from build123d import *

# Parameters (mm, degrees)
SKETCH1_R           = 32.5
BOSS_EXTRUDE1_DEPTH = 6
SKETCH16_R          = 1.1
CUT_EXTRUDE8_DEPTH  = 7
SKETCH17_R          = 2
CUT_EXTRUDE9_DEPTH  = 2.4
SKETCH12_R          = 1.65
CUT_EXTRUDE10_DEPTH = 7
CUT_EXTRUDE11_DEPTH = 3
CUT_EXTRUDE12_DEPTH = 7


with BuildPart() as part:
    # Sketch1 → Boss-Extrude1 (new body)
    with BuildSketch(Plane.XY):
        Circle(SKETCH1_R)
    extrude(amount=BOSS_EXTRUDE1_DEPTH)

    # Sketch16 → Cut-Extrude8 (cut, through all)
    with BuildSketch(Plane.XY.offset(6)):
        with Locations((8, 0)):
            Circle(SKETCH16_R)
        with Locations((-8, 0)):
            Circle(SKETCH16_R)
        with Locations((0, -8)):
            Circle(SKETCH16_R)
        with Locations((0, 8)):
            Circle(SKETCH16_R)
    extrude(amount=-CUT_EXTRUDE8_DEPTH, mode=Mode.SUBTRACT)

    # Sketch17 → Cut-Extrude9 (cut)
    with BuildSketch(Plane.XY.offset(6)):
        with Locations((8, 0)):
            Circle(SKETCH17_R)
        with Locations((-8, 0)):
            Circle(SKETCH17_R)
        with Locations((0, -8)):
            Circle(SKETCH17_R)
        with Locations((0, 8)):
            Circle(SKETCH17_R)
    extrude(amount=-CUT_EXTRUDE9_DEPTH, mode=Mode.SUBTRACT)

    # Sketch12 → Cut-Extrude10 (cut, through all)
    with BuildSketch(Plane.XY.offset(6)):
        with Locations((0, 28)):
            Circle(SKETCH12_R)
        with Locations((28, 0)):
            Circle(SKETCH12_R)
        with Locations((0, -28)):
            Circle(SKETCH12_R)
        with Locations((-28, 0)):
            Circle(SKETCH12_R)
    extrude(amount=-CUT_EXTRUDE10_DEPTH, mode=Mode.SUBTRACT)

    # Sketch18 → Cut-Extrude11 (cut)
    with BuildSketch(Plane(origin=(0, 0, 0), x_dir=(-1, 0, 0), z_dir=(0, 0, -1))):
        Polygon((1.616580754, 30.8), (-1.616580754, 30.8), (-3.233161507, 28), (-1.616580754, 25.2), (1.616580754, 25.2), (3.233161507, 28), align=None)
        Polygon((29.616580754, 2.8), (26.383419246, 2.8), (24.766838493, 0), (26.383419246, -2.8), (29.616580754, -2.8), (31.233161507, 0), align=None)
        Polygon((1.616580754, -25.2), (-1.616580754, -25.2), (-3.233161507, -28), (-1.616580754, -30.8), (1.616580754, -30.8), (3.233161507, -28), align=None)
        Polygon((-26.383419246, 2.8), (-29.616580754, 2.8), (-31.233161507, 0), (-29.616580754, -2.8), (-26.383419246, -2.8), (-24.766838493, 0), align=None)
    extrude(amount=-CUT_EXTRUDE11_DEPTH, mode=Mode.SUBTRACT)

    # Sketch19 → Cut-Extrude12 (cut, through all)
    with BuildSketch(Plane.XY.offset(6)):
        with BuildLine():
            ThreePointArc((12.212964584, -14.554844419), (0, 19), (-12.212964584, -14.554844419))
            ThreePointArc((-12.212964584, -14.554844419), (-7.986468426, -14.185073919), (-8.356238926, -9.958577761))
            ThreePointArc((-8.356238926, -9.958577761), (0, 13), (8.356238926, -9.958577761))
            ThreePointArc((8.356238926, -9.958577761), (7.986468426, -14.185073919), (12.212964584, -14.554844419))
        make_face()
    extrude(amount=-CUT_EXTRUDE12_DEPTH, mode=Mode.SUBTRACT)


solid = part.part
Design review of the part built by this model. Coordinates are the model's own, in mm. A direction names the side the tool comes from. Round coordinates to 2 decimals unless told otherwise and drop trailing zeros. Order: outer loops, then holes, each group sorted by start corner. A loop starts at its lowest first (then second) coordinate and runs counter-clockwise, first axis right, second up.
1) For L1, parallel to Y at x = 0, z = 2.9; L2, parallel to Y at x = 0, z = 3.7; L3, parallel to X at y = 2.5, z = 1.8, list the stretches that pass through material, from the lowest coordinate up.
The answers:
L1: y = -32.5 to -30.8, -25.2 to -9.1, -6.9 to 6.9, 9.1 to 13, 19 to 25.2, 30.8 to 32.5
L2: y = -32.5 to -29.65, -26.35 to -10, -6 to 6, 10 to 13, 19 to 26.35, 29.65 to 32.5
L3: x = -32.4 to -29.79, -26.21 to -18.83, -12.76 to 12.76, 18.83 to 26.21, 29.79 to 32.4
2) Clearance check with flat-ended pins moving along their axes: pin 1 Ø2.5 at (x, y) = (-8, 0) entering from -Z; pin 2 Ø1.5 at (x, z) = (0, 1) entering from -Y; pin 3 Ø1.5 at (x, z) = (27.5, 2) entering from +Y; pin 4 Ø3.5 at (x, z) = (28.5, 2) entering from -Y. State where each tip first meets the part, or that it passes through.
The answers:
pin 1: stops at z = 0
pin 2: stops at y = -32.5
pin 3: stops at y = 18.46
pin 4: stops at y = -18.46
3) Consider section C-C (z = 1.4). Count the separate pieces of the cut face and the enclosed holes in it, plus the area to 3 significant figures.
The answers:
separate pieces: 1
enclosed holes: 9
area: 2,700 mm2
4) Consider section A-A (x = -28). State the section outline as (y, z) points.
The answers:
outline: (-16.5, 0) - (-2.8, 0) - (-2.8, 3) - (-1.65, 3) - (-1.65, 6) - (-16.5, 6) - close; (1.65, 3) - (2.8, 3) - (2.8, 0) - (16.5, 0) - (16.5, 6) - (1.65, 6) - close
5) Consider section B-B (y = -4). State the section outline as (x, z) points, plus the area to 3 significant figures.
The answers:
outline: (-32.25, 0) - (-18.57, 0) - (-18.57, 6) - (-32.25, 6) - close; (-12.37, 0) - (12.37, 0) - (12.37, 6) - (-12.37, 6) - close; (18.57, 0) - (32.25, 0) - (32.25, 6) - (18.57, 6) - close
area: 313 mm2
6) Consider section D-D (y = 8). State the section outline as (x, z) points, plus the area to 3 significant figures.
The answers:
outline: (-31.5, 0) - (-17.23, 0) - (-17.23, 6) - (-31.5, 6) - close; (-10.25, 0) - (-1.1, 0) - (-1.1, 3.6) - (-2, 3.6) - (-2, 6) - (-10.25, 6) - close; (1.1, 0) - (10.25, 0) - (10.25, 6) - (2, 6) - (2, 3.6) - (1.1, 3.6) - close; (17.23, 0) - (31.5, 0) - (31.5, 6) - (17.23, 6) - close
area: 277 mm2
7) Machinability: for faces 1 (the flat face through (9, -1, 3.6)), 2 (the flat face through (-28, -2.8, 1)), 3 (the cylindrical face through (9.016, -0.421, 1.825)), which of the approach directions +Z, -Z, +X, -X, +Y, -Y give a long, thin tool a straight path to every point of the face, cutting with its end or side? Answer none if there is none.
The answers:
face 1: +Z
face 2: -Z
face 3: +Z, -Z
